from build123d import *

# Parameters (mm, degrees)
BOSS_EXTRUDE1_DEPTH                  = 60
FILLET1_R                            = 1
F_2_7_START                          = -7
F_2_7_2_7_DIAMETER_HOLE1_OUTLINE_R   = 1.35
F_2_7_2_7_DIAMETER_HOLE1_DEPTH       = 7
F_2_7_START_2                        = -8.6
F_2_7_2_7_DIAMETER_HOLE1_2_OUTLINE_R = 1.35
F_2_7_2_7_DIAMETER_HOLE1_2_DEPTH     = 1.6


# Read off the part's stored shape, not the designer's step: Ø2.7 (2.7) Diameter Hole1
with BuildPart() as part:
    # Sketch1 → Boss-Extrude1 (new body)
    with BuildSketch(Plane.XY):
        with BuildLine():
            Line((0, 0), (7.65, 0))
            Line((7.65, 0), (7.65, -1.6))
            ThreePointArc((7.65, -1.6), (15.413932023, -11.346794345), (26.65, -5.958898944))
            Line((26.65, -5.958898944), (28.65, -5.958898944))
            ThreePointArc((28.65, -5.958898944), (39.886067977, -11.346794345), (47.65, -1.6))
            Line((47.65, -1.6), (52.15, -1.6))
            ThreePointArc((52.15, -1.6), (59.913932023, -11.346794345), (71.15, -5.958898944))
            Line((71.15, -5.958898944), (73.15, -5.958898944))
            ThreePointArc((73.15, -5.958898944), (84.386067977, -11.346794345), (92.15, -1.6))
            Line((92.15, -1.6), (92.15, 0))
            Line((92.15, 0), (99.8, 0))
            Line((99.8, 0), (99.8, -1.6))
            Line((99.8, -1.6), (96.3, -1.6))
            Line((96.3, -1.6), (96.3, -7))
            Line((96.3, -7), (92.86634266, -7))
            ThreePointArc((92.86634266, -7), (84.043434268, -13.449679602), (73.65, -10.070537173))
            Line((73.65, -10.070537173), (70.65, -10.070537173))
            ThreePointArc((70.65, -10.070537173), (61.186027008, -13.561218837), (52.403205655, -8.6))
            Line((52.403205655, -8.6), (47.396794345, -8.6))
            ThreePointArc((47.396794345, -8.6), (38.613972992, -13.561218837), (29.15, -10.070537173))
            Line((29.15, -10.070537173), (26.15, -10.070537173))
            ThreePointArc((26.15, -10.070537173), (15.756565732, -13.449679602), (6.93365734, -7))
            Line((6.93365734, -7), (3.5, -7))
            Line((3.5, -7), (3.5, -1.6))
            Line((3.5, -1.6), (0, -1.6))
            Line((0, -1.6), (0, 0))
        make_face()
    extrude(amount=BOSS_EXTRUDE1_DEPTH)

    # Fillet1
    fillet1_edges = [part.edges().sort_by_distance(p)[0] for p in [
        (96.3, -1.6, 30),
        (92.86634266, -7, 30),
        (6.93365734, -7, 30),
        (3.5, -1.6, 30),
    ]]
    fillet(fillet1_edges, radius=FILLET1_R)

    # Ø2.7 (2.7) Diameter Hole1 outline → Ø2.7 (2.7) Diameter Hole1 (cut)
    with BuildSketch(Plane(origin=(0, 0, 0), x_dir=(1, 0, 0), z_dir=(0, 1, 0)).offset(F_2_7_START)):
        with Locations((94.4, -15)):
            Circle(F_2_7_2_7_DIAMETER_HOLE1_OUTLINE_R)
        with Locations((94.4, -45)):
            Circle(F_2_7_2_7_DIAMETER_HOLE1_OUTLINE_R)
        with Locations((49.9, -15)):
            Circle(F_2_7_2_7_DIAMETER_HOLE1_OUTLINE_R)
        with Locations((49.9, -45)):
            Circle(F_2_7_2_7_DIAMETER_HOLE1_OUTLINE_R)
    f_2_7_2_7_diameter_hole1 = extrude(amount=F_2_7_2_7_DIAMETER_HOLE1_DEPTH, mode=Mode.SUBTRACT)

    # 2.7 _2.7_ Diameter Hole1 2 outline → 2.7 _2.7_ Diameter Hole1 2 (cut)
    with BuildSketch(Plane(origin=(0, 0, 0), x_dir=(1, 0, 0), z_dir=(0, 1, 0)).offset(F_2_7_START_2)):
        with Locations((49.9, -15)):
            Circle(F_2_7_2_7_DIAMETER_HOLE1_2_OUTLINE_R)
        with Locations((49.9, -45)):
            Circle(F_2_7_2_7_DIAMETER_HOLE1_2_OUTLINE_R)
    f_2_7_2_7_diameter_hole1_2 = extrude(amount=F_2_7_2_7_DIAMETER_HOLE1_2_DEPTH, mode=Mode.SUBTRACT)

    # Mirror1: Ø2.7 (2.7) Diameter Hole1, 2.7 _2.7_ Diameter Hole1 2 across plane
    add(f_2_7_2_7_diameter_hole1.mirror(Plane.ZY.offset(-49.9)), mode=Mode.SUBTRACT)
    add(f_2_7_2_7_diameter_hole1_2.mirror(Plane.ZY.offset(-49.9)), mode=Mode.SUBTRACT)


solid = part.part
Read the model definition and answer for the solid it produces. Units are mm, in the model's axes. A direction names the side the tool comes from. Round coordinates to 2 decimals unless told otherwise and drop trailing zeros. Write each loop counter-clockwise with the first axis right and the second up, starting at its lowest first coordinate (ties: lowest second). Pieces come first, ordered by that corner, then holes.
1. Determine the mould class of faces 1 (the face through (15.231, -11.303, 29.58)), 2 (the face through (5.69, -3.55, 46.32)) for opening direction Z: pulls with the +Z half, pulls with the -Z half, needs draft (parallel to the pull), parting line crosses it, or undercut.
2. The part is cut by section A-A, the plane x = 49.9. Determine the outline of the cut face in (y, z), then the cut area to 3 significant figures.
3. Which of the six approach directions +Z, -Z, +X, -X, +Y, -Y give full straight-line access (tool end or side, diameter ignored) to faces 3 (the face through (28, -10.071, 30)), 4 (the face through (96.3, -5, 30)), 5 (the face through (50, -1.6, 30)), 6 (the face through (93.33, -3.55, 45.82)), 7 (the face through (1, -1.6, 30))?
4. Given pin 1 Ø4 at (y, z) = (-10, 30) entering from +X; pin 2 Ø4.5 at (x, z) = (5.4, 15) entering from -Y; pin 3 Ø6 at (y, z) = (-7, 20) entering from +X, each flat-ended and moving along its own axis, determine where each tip first touches the part or whether it passes through.
5. The part is cut by section B-B, the plane z = 45. State how many separate pieces and enclosed holes the cut face has, then the cut area to 3 significant figures.
6. Straight lines are drawn through the part: L1, parallel to Z at x = 5.4, y = -2; L2, parallel to X at y = -1.25, z = 15; L3, parallel to X at y = -5.5, z = 45. For each, find the intervals that lie inside material, in ascending order.
7. The part is cut by section D-D, the plane x = 13. Determine the outline of the cut face in (y, z).
Values:
1. face 1: needs draft
1. face 2: undercut
2. outline: (-8.6, 0) - (-1.6, 0) - (-1.6, 13.65) - (-8.6, 13.65) - close; (-8.6, 16.35) - (-1.6, 16.35) - (-1.6, 43.65) - (-8.6, 43.65) - close; (-8.6, 46.35) - (-1.6, 46.35) - (-1.6, 60) - (-8.6, 60) - close
2. area: 382 mm2
3. face 3: +Z, -Z, -Y
3. face 4: +Z, -Z, +X, -Y
3. face 5: +Z, -Z, +Y
3. face 6: +Y
3. face 7: +Z, -Z, -X, -Y
4. pin 1: stops at x = 92.3
4. pin 2: stops at y = -8.23
4. pin 3: stops at x = 96.3
5. separate pieces: 4
5. enclosed holes: 0
5. area: 250 mm2
6. L1: z = 0 to 13.65, 16.35 to 43.65, 46.35 to 60
6. L2: x = 0 to 4.05, 6.75 to 7.65, 92.15 to 93.05, 95.75 to 99.8
6. L3: x = 3.5 to 4.05, 6.75 to 8.44, 46.86 to 48.55, 51.25 to 52.94, 91.36 to 93.05, 95.75 to 96.3
7. outline: (-12.66, 0) - (-10.45, 0) - (-10.45, 60) - (-12.66, 60) - close
